Work out the finished part from the listing and answer in its coordinate system (mm). Face numbers are marked on the shaded views. A direction names the side the tool comes from. Give positions to 0.01 mm unless a question says otherwise; leave off trailing zeros. Loops run counter-clockwise (first coordinate to the right, second up) from the corner with the lowest first, then second, coordinate; pieces in that order, holes last. Notation, with made-up numbers: (41.25, 0) - (50.25, 0) arc R19 cw to (50.25, 32) - close; hole circle Ø3 at (75.5, 11). An arc over 180 degrees is marked (long way). One line per item, written item: value.
from build123d import *

# Parameters (mm, degrees)
CROQUIS1_R              = 19.05
SALIENTE_EXTRUIR1_DEPTH = 100
SALIENTE_EXTRUIR2_START = -15
SALIENTE_EXTRUIR2_DEPTH = 15


with BuildPart() as part:
    # Croquis1 → Saliente-Extruir1 (new body)
    with BuildSketch(Plane.XY):
        Circle(CROQUIS1_R)
    extrude(amount=SALIENTE_EXTRUIR1_DEPTH)

    # Croquis2 → Saliente-Extruir2 (add)
    with BuildSketch(Plane.XY.offset(100).offset(SALIENTE_EXTRUIR2_START)):
        with BuildLine():
            Line((19.05, 19.05), (0, 19.05))
            ThreePointArc((0, 19.05), (13.470384182, 13.470384182), (19.05, 0))
            Line((19.05, 0), (19.05, 19.05))
        make_face()
        with BuildLine():
            ThreePointArc((-19.05, 0), (-13.470384182, 13.470384182), (0, 19.05))
            Line((0, 19.05), (-19.05, 19.05))
            Line((-19.05, 19.05), (-19.05, 0))
        make_face()
    extrude(amount=SALIENTE_EXTRUIR2_DEPTH)


solid = part.part
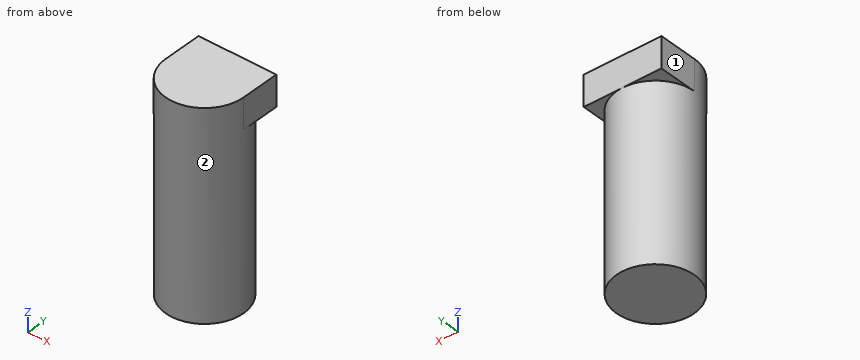
1. For the marked faces 1 and 2, determine the directions among +Z, -Z, +X, -X, +Y, -Y from which every point of the face is accessible in a straight line to the end or side of a thin tool.
Output:
face 1: +Z, -Z, -X, +Y, -Y
face 2: -Z
2. Find the intervals of material crossed by line 1 along Z through (x, y) = (-15.5, 11.5); line 2 along Y through (x, z) = (0, 56); line 3 along X through (y, z) = (9.5, 63), in increasing order.
Output:
line 1: z = 85 to 100
line 2: y = -19.05 to 19.05
line 3: x = -16.51 to 16.51
3. Section C-C (z = 90.5) is taken. Write down the section's boundary in (x, y), and give its area (3 significant figures).
Output:
outline: (-19.05, 0) arc R19.05 ccw to (19.05, 0) - (19.05, 19.05) - (-19.05, 19.05) - close
area: 1,300 mm²
4. Section B-B (y = 7.5) is taken. Write down the section's boundary in (x, z).
Output:
outline: (-19.05, 85) - (-17.51, 85) - (-17.51, 0) - (17.51, 0) - (17.51, 85) - (19.05, 85) - (19.05, 100) - (-19.05, 100) - close
5. Section A-A (x = 13) is taken. Write down the section's boundary in (y, z), and give its area (3 significant figures).
Output:
outline: (-13.92, 0) - (13.92, 0) - (13.92, 85) - (19.05, 85) - (19.05, 100) - (-13.92, 100) - close
area: 2,860 mm²
6. Section D-D (z = 55.5) is taken. Write down the section's boundary in (x, y).
Output:
outline: circle Ø38.1 at (0, 0)
7. Flat-ended cylindrical pins translate along their axes: pin 1 Ø2 at (x, z) = (-3, 43.5) entering from -Y; pin 2 Ø1.5 at (x, z) = (-10.5, 69) entering from -Y; pin 3 Ø8 at (y, z) = (-10, 79) entering from -X. Find the tip coordinate at first contact, or state that the pin passes through.
Output:
pin 1: stops at y = -18.94
pin 2: stops at y = -16.37
pin 3: stops at x = -18.08
